Autodesk Inventor part; units mm, degrees
ref_plane "YZ Plane" through (0, 0, 0) normal (1, 0, 0) x (0, 1, 0)
ref_plane "XZ Plane" through (0, 0, 0) normal (0, 1, 0) x (-1, 0, 0)
ref_plane "XY Plane" through (0, 0, 0) normal (0, 0, 1) x (1, 0, 0)
sketch "Sketch1" plane through (0, 0, 0) normal (0, 1, 0) x (-1, 0, 0)
  line L0 (58.83, 0) -> (0, 0)
  line L1 (0, 0) -> (0, -81.82)
  line L2 (0, -81.82) -> (58.83, -81.82)
  line L3 (58.83, -81.82) -> (58.83, 0)
  point P0 (0, 0)
  dimension "d0" = 58.83
  dimension "d1" = 81.82
extrude "Extrusion1" add sketch "Sketch1" along normal blind 1
sketch "Sketch2" plane through (0, 1, 0) normal (0, 1, 0) x (1, 0, 0)
  line L0 (-56.83, 0) -> (-58.83, 2)
  line L1 (-56.83, 81.82) -> (-58.83, 79.82)
  line L2 (0, 79.82) -> (-2, 81.82)
  line L3 (-2, 0) -> (0, 2)
  line L4 (-58.83, 0) -> (0, 0)
  line L5 (-58.83, 0) -> (-58.83, 2)
  line L6 (-58.83, 81.82) -> (-58.83, 0)
  line L7 (-58.83, 0) -> (-56.83, 0)
  line L8 (-58.83, 81.82) -> (-58.83, 79.82)
  line L9 (-58.83, 2) -> (-58.83, 0)
  line L10 (-58.83, 0) -> (-56.83, 0)
  line L11 (-2, 0) -> (0, 0)
  line L12 (0, 0) -> (0, 2)
  line L13 (0, 79.82) -> (0, 81.82)
  line L14 (0, 81.82) -> (-2, 81.82)
  line L15 (-56.83, 81.82) -> (-58.83, 81.82)
  dimension "d4" = 2
  dimension "d5" = 2
  dimension "d6" = 2
  dimension "d7" = 2
  dimension "d8" = 2
  dimension "d9" = 2
  dimension "d10" = 2
  dimension "d11" = 2
extrude "Extrusion2" add sketch "Sketch2" along normal blind 2.2
sketch "Sketch3" plane through (0, 0, 0) normal (0, -1, 0) x (1, 0, 0)
  line L0 (-58.83, 0) -> (0, 0)
  line L1 (-58.83, -81.82) -> (-58.83, 0)
  line L2 (0, -81.82) -> (-58.83, -81.82)
  line L3 (0, 0) -> (0, -81.82)
  line L4 (2, 2) -> (-60.83, 2)
  line L5 (-60.83, 2) -> (-60.83, -83.82)
  line L6 (-60.83, -83.82) -> (2, -83.82)
  line L7 (2, -83.82) -> (2, 2)
  point P0 (0, 0)
  dimension "d14" = 2
extrude "Extrusion3" add sketch "Sketch3" against normal blind 10.2
sketch "Sketch4" plane through (0, 10.2, 0) normal (0, 1, 0) x (1, 0, 0)
  line L0 (-58.83, 0) -> (-58.83, 81.82)
  line L1 (-58.83, 81.82) -> (0, 81.82)
  line L2 (0, 81.82) -> (0, 0)
  line L3 (0, 0) -> (-58.83, 0)
  line L4 (-60.83, -2) -> (2, -2)
  line L5 (2, -2) -> (2, 83.82)
  line L6 (2, 83.82) -> (-60.83, 83.82)
  line L7 (-60.83, 83.82) -> (-60.83, -2)
  line L8 (0, 0) -> (-2.3, 0)
  line L9 (-56.83, 0) -> (-2, 0)
  line L10 (2, -2) -> (-60.83, -2)
  line L11 (-2.3, 0) -> (-11.35, 0)
  line L12 (-11.35, 0) -> (-11.35, -2)
  line L13 (-11.35, -2) -> (-2.3, -2)
  line L14 (-2.3, -2) -> (-2.3, 0)
  point P0 (0, 0)
  dimension "d17" = 2.3
  dimension "d18" = 9.05
extrude "Extrusion4" cut sketch "Sketch4" against normal blind 7 contours L3 L14 L4 L12
sketch "Sketch5" plane through (0, 10.2, 0) normal (0, 1, 0) x (1, 0, 0)
  line L0 (0, 0) -> (0, 21.65)
  line L1 (0, 81.82) -> (0, 0)
  line L2 (2, -2) -> (2, 83.82)
  line L3 (0, 21.65) -> (2, 21.65)
  line L4 (2, 21.65) -> (2, 52.75)
  line L5 (2, 52.75) -> (0, 52.75)
  line L6 (0, 52.75) -> (0, 21.65)
  dimension "d21" = 21.65
  dimension "d22" = 31.1
extrude "Extrusion5" cut sketch "Sketch5" against normal blind 7
sketch "Sketch7" plane through (0, 3.2, -81.82) normal (-1, 0, 0) x (0, 0, 1)
  line L0 (60.17, 7) -> (60.17, 0)
  line L1 (60.17, 0) -> (29.07, 0)
  line L2 (29.07, 0) -> (29.07, 7)
  line L3 (0, 7) -> (29.07, 7)
  line L4 (2, -2.2) -> (2, 0)
  line L5 (79.82, -2.2) -> (2, -2.2)
  line L6 (79.82, -2.2) -> (79.82, 0)
  line L7 (81.82, 0) -> (79.82, 0)
  line L8 (81.82, 0) -> (81.82, 7)
  line L9 (60.17, 7) -> (81.82, 7)
  line L10 (0, 0) -> (0, 1.6)
  line L11 (0, 0) -> (0, 7)
  line L12 (0, 1.6) -> (13.65, 1.6)
  line L13 (29.07, 7) -> (29.07, 0)
  line L14 (13.65, 1.6) -> (29.07, 7)
  line L15 (29.07, 7) -> (-2, 7)
  line L16 (29.07, 7) -> (-2, 7)
  line L17 (-2, 7) -> (-2, 1.6)
  line L18 (-2, 1.6) -> (0, 1.6)
  point P0 (81.82, -3.2)
  dimension "d25" = 1.6
  dimension "d26" = 13.65
  dimension "d27" = 90
extrude "Extrusion6" cut sketch "Sketch7" against normal blind 7 and the other way blind 61 contours L3 L14 L12 L11
sketch "Sketch8" plane through (-60.83, 0, -83.82) normal (-1, 0, 0) x (0, 0, 1)
  line L0 (2, 4.8) -> (15.65, 4.8)
  line L1 (15.65, 4.8) -> (31.07, 10.2)
  line L2 (31.07, 10.2) -> (85.82, 10.2)
  line L3 (85.82, 10.2) -> (85.82, 0)
  line L4 (85.82, 0) -> (0, 0)
  line L5 (0, 0) -> (0, 10.2)
  line L6 (0, 10.2) -> (2, 10.2)
  line L7 (2, 10.2) -> (2, 4.8)
  line L8 (2, 4.8) -> (2, 10.2)
  line L9 (0, 10.2) -> (2, 10.2)
  line L10 (0, 0) -> (0, 10.2)
  line L11 (85.82, 0) -> (0, 0)
  line L12 (85.82, 0) -> (85.82, 10.2)
  line L13 (31.07, 10.2) -> (85.82, 10.2)
  line L14 (31.07, 10.2) -> (15.65, 4.8)
  line L15 (15.65, 4.8) -> (2, 4.8)
  line L16 (0, 10.2) -> (2, 10.2)
  line L17 (0, 10.2) -> (2, 10.2)
  line L18 (2, 10.2) -> (2, 4.8)
  line L19 (2, 4.8) -> (0, 4.8)
  line L20 (0, 4.8) -> (0, 10.2)
  point P0 (83.82, 0)
extrude "Extrusion7" cut sketch "Sketch8" against normal blind 63 contours L19 L5 L6 L7
sketch "Sketch9" plane through (0, 3.2, 0) normal (0, 1, 0) x (1, 0, 0)
  line L0 (-11.35, 0) -> (-2.3, 0)
  line L1 (-11.35, -2) -> (-11.35, 0)
  line L2 (-2.3, -2) -> (-11.35, -2)
  line L3 (-2.3, 0) -> (-2.3, -2)
  line L4 (2, 21.65) -> (0, 21.65)
  line L5 (2, 52.75) -> (2, 21.65)
  line L6 (0, 52.75) -> (2, 52.75)
  line L7 (0, 21.65) -> (0, 52.75)
  point P0 (0, 0)
extrude "Extrusion8" add sketch "Sketch9" along normal blind 1.6
equation "\"d5\" = d4"
equation "\"d6\" = d4"
equation "\"d7\" = d6"
properties part number "Enclosure"
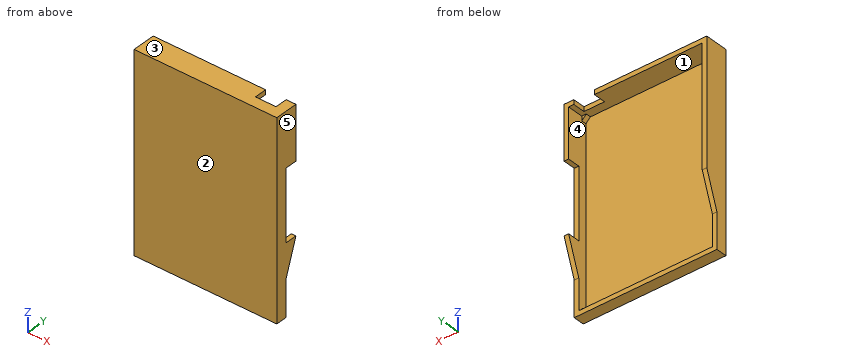
Geometry: final body of the model. Coordinates: model frame, mm. Face numbers are marked on the shaded views. A direction names the side the tool comes from. Give positions to 0.01 mm unless a question says otherwise; leave off trailing zeros. Write each loop counter-clockwise with the first axis right and the second up, starting at its lowest first coordinate (ties: lowest second). Pieces come first, ordered by that corner, then holes.
(1) Cut plane A-A, the plane y = 7.5. Return loops of the section in (x, z), then the cut area to 3 significant figures.
(2) Access query for the marked faces 1 and 2. Directions: +Z, -Z, +X, -X, +Y, -Y. A direction counts if a zero-diameter tool reaches every point of the face in a straight line with its end or side. Return the directions, or none.
(3) First-contact query: P1, Ø2, axis at x = -57.5, z = -80.5, coming from the +Y side; P2, Ø17.5, axis at x = -34, z = -33.5, coming from the +Y side; P3, Ø2, axis at x = 1.5, z = -38.5, coming from the +Y side. Flat tips, straight axial feed; report the tip coordinate or a pass-through.
(4) Cut plane B-B, the plane x = -8. Return loops of the section in (y, z), then the cut area to 3 significant figures.
(5) Ray query, line 1 (X direction, y = 8.5, z = -12); line 2 (Z direction, x = -27, y = 3); line 3 (Y direction, x = -35, z = -4.5). Return the intervals inside material, ascending.
(6) Mould query, pull axis Z, two halves, no side actions, for the marked faces 3, 4 and 5. Classes: released by +Z, released by -Z, zero draft, split by the parting line, or undercut.
(7) Cut plane C-C, the plane z = -6. Return loops of the section in (x, y).
Values follow:
1. outline: (-60.83, -60.46) - (-58.83, -60.46) - (-58.83, 0) - (-11.35, 0) - (-11.35, 2) - (-60.83, 2) - close; (-2.3, 0) - (0, 0) - (0, -21.65) - (2, -21.65) - (2, 2) - (-2.3, 2) - close; (0, -60.46) - (2, -60.46) - (2, -52.75) - (0, -52.75) - close
1. area: 287 mm2
2. face 1: +Y
2. face 2: +Z, -Z, +X, -X, -Y
3. P1: stops at y = 3.2
3. P2: stops at y = 1
3. P3: stops at y = 4.8
4. outline: (0, -83.82) - (4.8, -83.82) - (4.8, -81.82) - (1, -81.82) - (1, 0) - (4.8, 0) - (4.8, 2) - (0, 2) - close
4. area: 101 mm2
5. line 1: x = -60.83 to -58.83, 0 to 2
5. line 2: z = -83.82 to -81.82, 0 to 2
5. line 3: y = 0 to 1
6. face 3: released by +Z
6. face 4: undercut
6. face 5: zero draft
7. outline: (-60.83, 0) - (2, 0) - (2, 10.2) - (0, 10.2) - (0, 1) - (-58.83, 1) - (-58.83, 10.2) - (-60.83, 10.2) - close
